from build123d import *

# Parameters (mm, degrees)
SKETCH1_W                                       = 92
SKETCH1_H                                       = 92
BOSS_EXTRUDE1_DEPTH                             = 0.85
SKETCH2_W                                       = 72
SKETCH2_H                                       = 72
BOSS_EXTRUDE2_DEPTH                             = 2.3
CSK_FOR_M3_FLAT_HEAD_MACHINE_SCREW1_D           = 3.4
CSK_FOR_M3_FLAT_HEAD_MACHINE_SCREW1_CSINK_D     = 6.3
CSK_FOR_M3_FLAT_HEAD_MACHINE_SCREW1_CSINK_ANGLE = 90
FILLET1_R                                       = 2


with BuildPart() as part:
    # Sketch1 → Boss-Extrude1 (new, symmetric)
    with BuildSketch(Plane(origin=(0, 0, 0), x_dir=(1, 0, 0), z_dir=(0, 1, 0))):
        Rectangle(SKETCH1_W, SKETCH1_H)
    extrude(amount=BOSS_EXTRUDE1_DEPTH, both=True)

    # Sketch2 → Boss-Extrude2 (add)
    with BuildSketch(Plane(origin=(0, 0.85, 0), x_dir=(1, 0, 0), z_dir=(0, 1, 0))):
        Rectangle(SKETCH2_W, SKETCH2_H)
    extrude(amount=BOSS_EXTRUDE2_DEPTH)

    # CSK for M3 Flat Head Machine Screw1 (through all)
    with Locations(Plane(origin=(-41, -0.85, 41), x_dir=(0, 0, -1), z_dir=(0, -1, 0))):
        with Locations((0, 0), (0, 41), (0, 82), (41, 82), (82, 82), (82, 41), (82, 0), (41, 0)):
            CounterSinkHole(CSK_FOR_M3_FLAT_HEAD_MACHINE_SCREW1_D / 2, CSK_FOR_M3_FLAT_HEAD_MACHINE_SCREW1_CSINK_D / 2, counter_sink_angle=CSK_FOR_M3_FLAT_HEAD_MACHINE_SCREW1_CSINK_ANGLE)

    # Fillet1
    fillet1_edges = [part.edges().sort_by_distance(p)[0] for p in [
        (36, 2, 36),
        (36, 2, -36),
        (-36, 2, -36),
        (-36, 2, 36),
        (46, 0, 46),
        (-46, 0, 46),
        (-46, 0, -46),
        (46, 0, -46),
    ]]
    fillet(fillet1_edges, radius=FILLET1_R)


solid = part.part
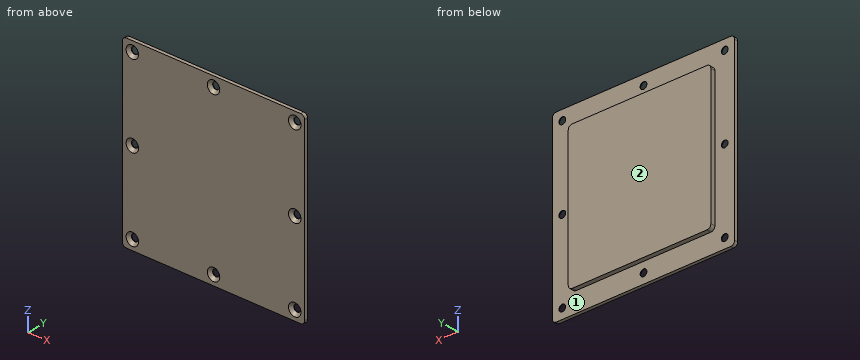
Geometry: final body of the model. Coordinates: model frame, mm. Face numbers are marked on the shaded views. A direction names the side the tool comes from. Round coordinates to 2 decimals unless told otherwise and drop trailing zeros. Order: outer loops, then holes, each group sorted by start corner. A loop starts at its lowest first (then second) coordinate and runs counter-clockwise, first axis right, second up. Notation, with made-up numbers: (-8, 76) -> (19, 76) arc R20 cw to (19, 110) -> close; hole circle Ø11 at (-27.75, 70). An arc over 180 degrees is marked (long way). Put each result on its own line as item: value. Start each with the question number.
Q1. First-contact query: pin 1 (1.8 mm diameter, centred on y = 2, z = -5, fed in from +X); pin 2 (2 mm diameter, centred on x = 41, z = 41, fed in from +Y) (3 decimals); pin 3 (4.5 mm diameter, centred on x = -41, z = 0, fed in from +Y); pin 4 (2 mm diameter, centred on x = -14.5, y = 2, fed in from +Z). Flat tips, straight axial feed; report the tip coordinate or a pass-through.
Q2. Section A-A on z = 0. Return the cut outline in (x, y), and give its area (3 significant figures).
Q3. Section C-C on z = -41. Return the cut outline in (x, y), and give its area (3 significant figures).
Q4. Section B-B on x = 41. Return the cut outline in (y, z).
Q5. Section D-D on y = 2.25. Return the cut outline in (x, z).
Q6. Reachability of the marked faces 1 and 2 from +Z, -Z, +X, -X, +Y, -Y: full face, straight path, thin tool, end or side. Return the list, or none.
Q7. Line query: probe 1 along X at (y, z) = (0.8, 0); probe 2 along X at (y, z) = (0.75, 41). Output: solid intervals per line, ascending.
Ans:
1. pin 1: stops at x = 36
1. pin 2: passes through
1. pin 3: stops at y = 0.85
1. pin 4: stops at z = 36
2. outline: (-46, -0.85) -> (-44.15, -0.85) -> (-42.7, 0.6) -> (-42.7, 0.85) -> (-46, 0.85) -> close; (-39.3, 0.6) -> (-37.85, -0.85) -> (37.85, -0.85) -> (39.3, 0.6) -> (39.3, 0.85) -> (36, 0.85) -> (36, 3.15) -> (-36, 3.15) -> (-36, 0.85) -> (-39.3, 0.85) -> close; (42.7, 0.6) -> (44.15, -0.85) -> (46, -0.85) -> (46, 0.85) -> (42.7, 0.85) -> close
2. area: 306 mm2
3. outline: (-46, -0.85) -> (-44.15, -0.85) -> (-42.7, 0.6) -> (-42.7, 0.85) -> (-46, 0.85) -> close; (-39.3, 0.6) -> (-37.85, -0.85) -> (-3.15, -0.85) -> (-1.7, 0.6) -> (-1.7, 0.85) -> (-39.3, 0.85) -> close; (1.7, 0.6) -> (3.15, -0.85) -> (37.85, -0.85) -> (39.3, 0.6) -> (39.3, 0.85) -> (1.7, 0.85) -> close; (42.7, 0.6) -> (44.15, -0.85) -> (46, -0.85) -> (46, 0.85) -> (42.7, 0.85) -> close
3. area: 133 mm2
4. outline: (-0.85, -46) -> (0.85, -46) -> (0.85, -42.7) -> (0.6, -42.7) -> (-0.85, -44.15) -> close; (-0.85, -37.85) -> (0.6, -39.3) -> (0.85, -39.3) -> (0.85, -1.7) -> (0.6, -1.7) -> (-0.85, -3.15) -> close; (-0.85, 3.15) -> (0.6, 1.7) -> (0.85, 1.7) -> (0.85, 39.3) -> (0.6, 39.3) -> (-0.85, 37.85) -> close; (-0.85, 44.15) -> (0.6, 42.7) -> (0.85, 42.7) -> (0.85, 46) -> (-0.85, 46) -> close
5. outline: (-36, -34) arc R2 ccw to (-34, -36) -> (34, -36) arc R2 ccw to (36, -34) -> (36, 34) arc R2 ccw to (34, 36) -> (-34, 36) arc R2 ccw to (-36, 34) -> close
6. face 1: +Y
6. face 2: +Z, -Z, +X, -X, +Y
7. probe 1: x = -46 to -42.7, -39.3 to 39.3, 42.7 to 46
7. probe 2: x = -46 to -42.7, -39.3 to -1.7, 1.7 to 39.3, 42.7 to 46
